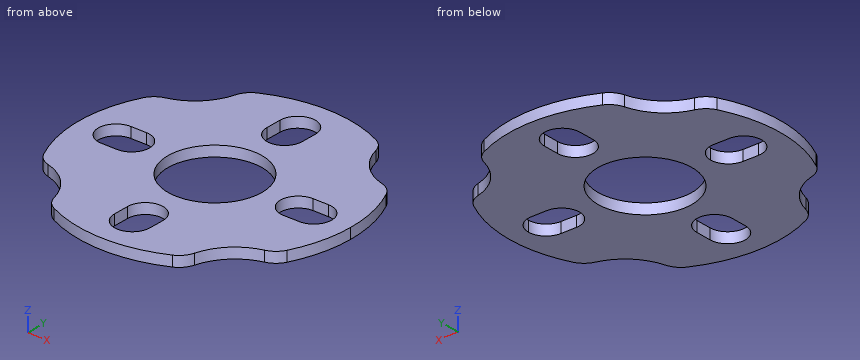
from build123d import *

# Parameters (mm, degrees)
F2_R     = 4.5
F3_DEPTH = 1
F4_R     = 2


with BuildPart() as f3:
    # F2 (on Top) → F3 (new body)
    with BuildSketch(Plane.XY):
        with BuildLine():
            ThreePointArc((11.2, -6.6), (12.5419296761, -3.4205262753), (13, 0))
            ThreePointArc((13, 0), (12.5419296761, 3.4205262753), (11.2, 6.6))
            ThreePointArc((11.2, 6.6), (8.0806476452, 8.0806476452), (6.6, 11.2))
            ThreePointArc((6.6, 11.2), (0, 13), (-6.6, 11.2))
            ThreePointArc((-6.6, 11.2), (-8.0806476452, 8.0806476452), (-11.2, 6.6))
            ThreePointArc((-11.2, 6.6), (-13, 0), (-11.2, -6.6))
            ThreePointArc((-11.2, -6.6), (-8.0806476452, -8.0806476452), (-6.6, -11.2))
            ThreePointArc((-6.6, -11.2), (0, -13), (6.6, -11.2))
            ThreePointArc((6.6, -11.2), (8.0806476452, -8.0806476452), (11.2, -6.6))
        make_face()
        with BuildLine():
            ThreePointArc((-1.7, -8), (0, -6.3), (1.7, -8))
            Line((1.7, -8), (1.7, -9.5))
            ThreePointArc((1.7, -9.5), (0, -11.2), (-1.7, -9.5))
            Line((-1.7, -9.5), (-1.7, -8))
        make_face(mode=Mode.SUBTRACT)
        with BuildLine():
            ThreePointArc((-9.5, -1.7), (-11.2, 0), (-9.5, 1.7))
            Line((-9.5, 1.7), (-8, 1.7))
            ThreePointArc((-8, 1.7), (-6.797918472, 1.202081528), (-6.3, 0))
            ThreePointArc((-6.3, 0), (-6.797918472, -1.202081528), (-8, -1.7))
            Line((-8, -1.7), (-9.5, -1.7))
        make_face(mode=Mode.SUBTRACT)
        Circle(F2_R, mode=Mode.SUBTRACT)
        with BuildLine():
            ThreePointArc((8, -1.7), (6.3, 0), (8, 1.7))
            Line((8, 1.7), (9.5, 1.7))
            ThreePointArc((9.5, 1.7), (10.702081528, 1.202081528), (11.2, 0))
            ThreePointArc((11.2, 0), (10.702081528, -1.202081528), (9.5, -1.7))
            Line((9.5, -1.7), (8, -1.7))
        make_face(mode=Mode.SUBTRACT)
        with BuildLine():
            ThreePointArc((-1.7, 9.5), (0, 11.2), (1.7, 9.5))
            Line((1.7, 9.5), (1.7, 8))
            ThreePointArc((1.7, 8), (0, 6.3), (-1.7, 8))
            Line((-1.7, 8), (-1.7, 9.5))
        make_face(mode=Mode.SUBTRACT)
    extrude(amount=F3_DEPTH)

    # F4
    f4_edges = [f3.edges().sort_by_distance(p)[0] for p in [
        (-11.2, -6.6, 0.5),
        (11.2, -6.6, 0.5),
        (11.2, 6.6, 0.5),
        (-11.2, 6.6, 0.5),
        (6.6, -11.2, 0.5),
        (-6.6, -11.2, 0.5),
        (-6.6, 11.2, 0.5),
        (6.6, 11.2, 0.5),
    ]]
    fillet(f4_edges, radius=F4_R)


solid = f3.part
The model under review builds one solid part; all positions refer to its coordinate system, in mm. Give positions to 0.01 mm unless a question says otherwise; leave off trailing zeros. Write each loop counter-clockwise with the first axis right and the second up, starting at its lowest first coordinate (ties: lowest second). Pieces come first, ordered by that corner, then holes.
1. Add section B-B, the plane y = 0.5. Write out the cut boundary in (x, z), plus the area to 3 significant figures.
2. Add section A-A, the plane x = 0. Write out the cut boundary in (y, z).
3. Wall thickness on L1, parallel to Y at x = 0, z = 0.35; L2, parallel to X at y = 0.75, z = 0.1; L3, parallel to X at y = 3, z = 0.7: over which ranges is each line inside the solid? List them lowest first.
4. Add section D-D, the plane y = 3.25. Write out the cut boundary in (x, z), plus the area to 3 significant figures.
5. Add section C-C, the plane x = -7.25. Write out the cut boundary in (y, z), plus the area to 3 significant figures.
6. For P1, Ø12, axis at x = -8.5, y = -8, coming from the +Z side; P2, Ø0.5, axis at y = 9, z = 0.5, coming from the +X side, all flat-tipped, find the tip position at first contact; note any pin that passes through.
Worked answers:
1. outline: (-12.99, 0) - (-11.12, 0) - (-11.12, 1) - (-12.99, 1) - close; (-6.38, 0) - (-4.47, 0) - (-4.47, 1) - (-6.38, 1) - close; (4.47, 0) - (6.38, 0) - (6.38, 1) - (4.47, 1) - close; (11.12, 0) - (12.99, 0) - (12.99, 1) - (11.12, 1) - close
1. area: 7.54 mm2
2. outline: (-13, 0) - (-11.2, 0) - (-11.2, 1) - (-13, 1) - close; (-6.3, 0) - (-4.5, 0) - (-4.5, 1) - (-6.3, 1) - close; (4.5, 0) - (6.3, 0) - (6.3, 1) - (4.5, 1) - close; (11.2, 0) - (13, 0) - (13, 1) - (11.2, 1) - close
3. L1: y = -13 to -11.2, -6.3 to -4.5, 4.5 to 6.3, 11.2 to 13
3. L2: x = -12.98 to -11.03, -6.47 to -4.44, 4.44 to 6.47, 11.03 to 12.98
3. L3: x = -12.65 to -3.35, 3.35 to 12.65
4. outline: (-12.59, 0) - (-3.11, 0) - (-3.11, 1) - (-12.59, 1) - close; (3.11, 0) - (12.59, 0) - (12.59, 1) - (3.11, 1) - close
4. area: 18.9 mm2
5. outline: (-9.17, 0) - (-1.53, 0) - (-1.53, 1) - (-9.17, 1) - close; (1.53, 0) - (9.17, 0) - (9.17, 1) - (1.53, 1) - close
5. area: 15.3 mm2
6. P1: stops at z = 1
6. P2: stops at x = 7.52
